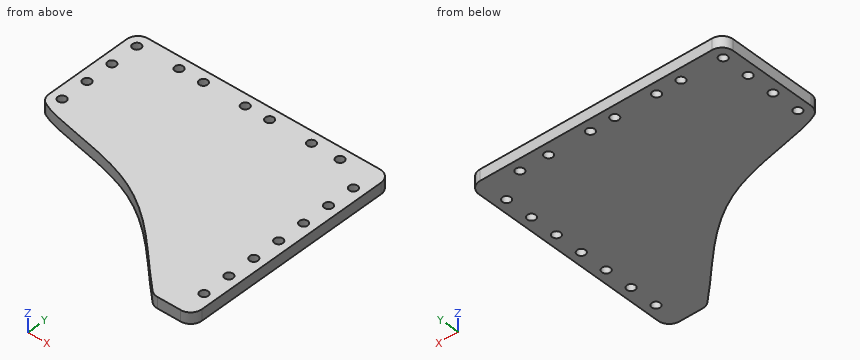
from build123d import *

# Parameters (mm, degrees)
F1_DEPTH = 5.08
F2_R     = 5.08
F2_R_2   = 5.07999
F3_R     = 1.905
F4_DEPTH = 5.0810001


# Not quite as in the source:
# - a fillet or chamfer is up to 0.001 mm smaller than in the source, because OpenCascade refuses the exact size


with BuildPart() as f1:
    # F0 (on Top) → F1 (new body)
    with BuildSketch(Plane.XY):
        with BuildLine():
            Line((-70.1164795637, 40.014226675), (-70.1164795637, -7.2926129862))
            add(Edge.make_bspline(
                [(-70.1164795637, -7.2926129862), (-65.04872861, -13.3058879533), (-12.1612328693, -14.8475963345), (11.7038576667, -47.1047081721), (28.178319335, -61.585773325)],
                knots=[0, 0, 0, 0, 0.4703732395, 1, 1, 1, 1], degree=3))
            Line((28.178319335, -61.585773325), (45.7710204363, -61.585773325))
            Line((45.7710204363, -61.585773325), (45.7710204363, 40.014226675))
            Line((45.7710204363, 40.014226675), (-70.1164795637, 40.014226675))
        make_face()
    extrude(amount=F1_DEPTH)

    # F2 (call 1 of 5: OpenCascade refuses the feature's edges together)
    f2_edges = [f1.edges().sort_by_distance(p)[0] for p in [
        (-70.11648, 40.014227, 2.54),
    ]]
    fillet(f2_edges, radius=F2_R)

    # F2#2 (call 2 of 5)
    f2_2_edges = [f1.edges().sort_by_distance(p)[0] for p in [
        (45.77102, 40.014227, 2.54),
    ]]
    fillet(f2_2_edges, radius=F2_R)

    # F2#4 (call 3 of 5)
    f2_4_edges = [f1.edges().sort_by_distance(p)[0] for p in [
        (28.178319, -61.585773, 2.54),
    ]]
    fillet(f2_4_edges, radius=F2_R)

    # F2#5 (call 4 of 5)
    f2_5_edges = [f1.edges().sort_by_distance(p)[0] for p in [
        (45.77102, -61.585773, 2.54),
    ]]
    fillet(f2_5_edges, radius=F2_R)

    # F2#3 (call 5 of 5) (radius 5.08 in the source; OpenCascade refuses exactly that, so slightly less here)
    f2_3_edges = [f1.edges().sort_by_distance(p)[0] for p in [
        (-70.11648, -7.292613, 2.54),
    ]]
    fillet(f2_3_edges, radius=F2_R_2)

    # F3 (on face) → F4 (cut, through all)
    with BuildSketch(Plane.XY.offset(5.08)):
        with Locations((-46.3039795637, 34.934226675)):
            Circle(F3_R)
        with Locations((-35.1914795637, 34.934226675)):
            Circle(F3_R)
        with Locations((-16.1414795637, 34.934226675)):
            Circle(F3_R)
        with Locations((-5.0289795637, 34.934226675)):
            Circle(F3_R)
        with Locations((14.0210204363, 34.934226675)):
            Circle(F3_R)
        with Locations((-65.0364795637, 34.3525031737)):
            Circle(F3_R)
        with Locations((-65.0364795637, 21.6525031737)):
            Circle(F3_R)
        with Locations((-65.0364795637, 8.9525031737)):
            Circle(F3_R)
        with Locations((-65.0364795637, -3.7474968263)):
            Circle(F3_R)
        with Locations((27.0512204363, 34.934226675)):
            Circle(F3_R)
        with Locations((40.6910204363, 26.4864852548)):
            Circle(F3_R)
        with Locations((40.6910204363, 13.7864852548)):
            Circle(F3_R)
        with Locations((40.6910204363, 1.0864852548)):
            Circle(F3_R)
        with Locations((40.6910204363, -11.6135147452)):
            Circle(F3_R)
        with Locations((40.6910204363, -24.3135147452)):
            Circle(F3_R)
        with Locations((40.6910204363, -37.0135147452)):
            Circle(F3_R)
        with Locations((40.6910204363, -49.7135147452)):
            Circle(F3_R)
    extrude(amount=-F4_DEPTH, mode=Mode.SUBTRACT)


solid = f1.part
The model under review builds one solid part; all positions refer to its coordinate system, in mm. Coordinates: 2 decimals unless noted, no trailing zeros. Use a Markdown table: item, result. Add a question column.
1. To check wall thickness, follow line 1 (Y direction, x = -64, z = 2.45); line 2 (X direction, y = 20.5, z = 4.6); line 3 (X direction, y = 15, z = 4.5). State the ranges of each line that lie inside material, in increasing order.
2. Clearance check with flat-ended pins moving along their axes: pin 1 Ø2.5 at (x, y) = (-65.04, 8.95) entering from -Z; pin 2 Ø3 at (x, z) = (-56.5, 3) entering from -Y. State where each tip first meets the part, or that it passes through.
3. Add section A-A on z = 2.75. Give the number of separate pieces and of enclosed holes in the cut face, plus the area to 3 significant figures.
Returned:
| question | item | result |
|---|---|---|
| 1 | line 1 | y = -10.68 to -5.35, -2.15 to 7.35, 10.55 to 20.05, 23.25 to 32.75, 35.95 to 40.01 |
| 1 | line 2 | x = -70.12 to -66.55, -63.52 to 45.77 |
| 1 | line 3 | x = -70.12 to 39.22, 42.16 to 45.77 |
| 2 | pin 1 | passes through |
| 2 | pin 2 | stops at y = -13.01 |
| 3 | separate pieces | 1 |
| 3 | enclosed holes | 17 |
| 3 | area | 8,190 mm² |
